from build123d import *

# Parameters (mm, degrees)
SKETCH1_R           = 3.175
EXTRUDE1_DEPTH      = 44.45
SKETCH2_R           = 4.826
EXTRUDE2_DEPTH      = 2.54
CHAMFER1_SIZE       = 0.508
SKETCH3_R           = 1.190625
EXTRUDE3_DEPTH      = 5.826
EXTRUDE3_DEPTH_BACK = 5.826
CHAMFER2_SIZE       = 0.3175


with BuildPart() as part:
    # Sketch1 → Extrude1 (new body, symmetric)
    with BuildSketch(Plane.XY):
        Circle(SKETCH1_R)
    extrude(amount=EXTRUDE1_DEPTH, both=True)

    # Sketch2 → Extrude2 (add)
    with BuildSketch(Plane.XY.offset(44.45)):
        Circle(SKETCH2_R)
    extrude(amount=EXTRUDE2_DEPTH)

    # Chamfer1
    chamfer1_edges = [part.edges().sort_by_distance(p)[0] for p in [
        (-4.826, 0, 46.99),
    ]]
    chamfer(chamfer1_edges, length=CHAMFER1_SIZE)

    # Sketch3 → Extrude3 (cut, two sides)
    with BuildSketch(Plane(origin=(0, 0, 0), x_dir=(0, 0, -1), z_dir=(1, 0, 0))) as extrude3_sk:
        with Locations((40.878125, 0)):
            Circle(SKETCH3_R)
    extrude(amount=EXTRUDE3_DEPTH, mode=Mode.SUBTRACT)
    extrude(extrude3_sk.sketch, amount=-EXTRUDE3_DEPTH_BACK, mode=Mode.SUBTRACT)

    # Chamfer2
    chamfer2_edges = [part.edges().sort_by_distance(p)[0] for p in [
        (-3.175, 0, -44.45),
    ]]
    chamfer(chamfer2_edges, length=CHAMFER2_SIZE)


solid = part.part
CAD build for the part. Positions are in the model's coordinates, mm. A direction names the side the tool comes from. Round coordinates to 2 decimals unless told otherwise and drop trailing zeros. Order: outer loops, then holes, each group sorted by start corner. A loop starts at its lowest first (then second) coordinate and runs counter-clockwise, first axis right, second up. Notation, with made-up numbers: (57.25, 6) -> (85.25, 6) arc R12 cw to (85.25, 13) -> close; hole circle Ø9 at (11, -0.5). An arc over 180 degrees is marked (long way). Write each question's results on one line, items separated by ' | '.
1. Cut at B-B (z = -33.5). Give the cut face in (x, y) (3 decimals), plus the area to 3 significant figures.
Findings below:
outline: circle Ø6.35 at (0, 0) | area: 31.7 mm²
2. Flat gauge pins, fed straight in: P1, Ø1, axis at y = -2.5, z = -32, coming from the -X side; P2, Ø1, axis at y = 0, z = 23.5, coming from the -X side (3 decimals); P3, Ø1.5, axis at x = 2, z = 8.5, coming from the -Y side. Where does each tip first touch, or does it go through?
Findings below:
P1: stops at x = -2.47 | P2: stops at x = -3.175 | P3: stops at y = -2.92
3. Wall check: line 1 along Z through (x, y) = (2.2, 0); line 2 along Y through (x, z) = (0.25, 16.5); line 3 along Z through (x, y) = (4.25, -0.25). Give the ranges that are in metal, low to high. Write a range as [from, to].
Findings below:
line 1: z = [-44.45, -42.07], [-39.69, 46.99] | line 2: y = [-3.17, 3.17] | line 3: z = [44.45, 46.99]
4. 3-axis set-ups, long thin cutter, end or side, ignore diameter. For faces 1 (the face through (0, 0, -44.45)), 2 (the face through (-0.69, -3.1, 0.78)): which of +Z, -Z, +X, -X, +Y, -Y reach the whole face in a straight line?
Findings below:
face 1: -Z, +X, -X, +Y, -Y | face 2: -Z
